Can you work these out from the model? Positions are in its coordinate system, mm. A direction names the side the tool comes from. Give positions to 0.01 mm unless a question says otherwise; leave off trailing zeros. Loops run counter-clockwise (first coordinate to the right, second up) from the corner with the lowest first, then second, coordinate; pieces in that order, holes last. Notation, with made-up numbers: (-36.5, 4.25) - (12.5, 4.25) arc R33 ccw to (12.5, 33.25) - close; hole circle Ø3 at (67, 45.5). An arc over 180 degrees is marked (long way). Write item = value, one per line.
from build123d import *

# Parameters (mm, degrees)
F1_DEPTH  = 9
F2_W      = 42.22
F2_H      = 1.875
F3_DEPTH  = 1
F4_W      = 10
F4_H      = 9
F5_DEPTH  = 10
F6_R      = 9.99999
F7_R      = 4.5
F8_DEPTH  = 25
F10_DEPTH = 5
F12_DEPTH = 25


# Not quite as in the source:
# - a fillet or chamfer is up to 0.001 mm smaller than in the source, because OpenCascade refuses the exact size


with BuildPart() as f1:
    # F0 (on Front) → F1 (new body)
    with BuildSketch(Plane.XZ):
        Polygon((30, 3.7309644414), (0, 3.7309644414), (-30, 3.7309644414), (-40, 18.7309644414), (-45, 18.7309644414), (-40, -1.2690355586), (-45, -11.2690355586), (-30, -6.2690355586), (0, -6.2690355586), (30, -6.2690355586), (45, -11.2690355586), (40, -1.2690355586), (45, 18.7309644414), (40, 18.7309644414), align=None)
    extrude(amount=F1_DEPTH)

    # F2 (on face) → F3 (cut)
    with BuildSketch(Plane.XY.offset(3.7309644414)):
        Polygon((21.11, -8.25), (25, -4.5), (21.11, -4.5), (21.11, -6.375), align=None)
        Polygon((21.11, -4.5), (25, -4.5), (21.11, -0.75), (21.11, -2.625), align=None)
        with Locations((0, -5.4375)):
            Rectangle(F2_W, F2_H)
        with Locations((0, -3.5625)):
            Rectangle(F2_W, F2_H)
        Polygon((-21.11, -6.375), (-21.11, -4.5), (-25, -4.5), (-21.11, -8.25), align=None)
        Polygon((-25, -4.5), (-21.11, -4.5), (-21.11, -2.625), (-21.11, -0.75), align=None)
    extrude(amount=-F3_DEPTH, mode=Mode.SUBTRACT)

    # F4 (on face) → F5 (join)
    with BuildSketch(Plane(origin=(0, 0, -6.2690355586), x_dir=(1, 0, 0), z_dir=(0, 0, -1))):
        with Locations((0, 4.5)):
            Rectangle(F4_W, F4_H)
    extrude(amount=F5_DEPTH)

    # F6 (radius 10 in the source; OpenCascade refuses exactly that, so slightly less here)
    f6_edges = [f1.edges().sort_by_distance(p)[0] for p in [
        (5, -4.5, -6.269036),
        (-5, -4.5, -6.269036),
    ]]
    fillet(f6_edges, radius=F6_R)

    # F7 (on face) → F8 (join)
    with BuildSketch(Plane(origin=(0, 0, -16.2690355586), x_dir=(1, 0, 0), z_dir=(0, 0, -1))):
        with Locations((0, 4.5)):
            Circle(F7_R)
    extrude(amount=F8_DEPTH)

    # F9 (on face) → F10 (join)
    with BuildSketch(Plane(origin=(0, 0, -41.2690355586), x_dir=(1, 0, 0), z_dir=(0, 0, -1))):
        Polygon((-10, 0), (0, 0), (10.0785335526, 0), (10.0785335526, 9), (0, 9), (-10, 9), align=None)
    extrude(amount=F10_DEPTH)

    # F11 (on face) → F12 (cut)
    with BuildSketch(Plane.XZ.offset(9)):
        Polygon((-10, -41.2690355586), (-10, -42.9390355586), (-4.5407158323, -41.2690355586), align=None)
        Polygon((10.0785335526, -41.2690355586), (4.5102024451, -41.2690355586), (10.0785335526, -42.9390355586), align=None)
    extrude(amount=-F12_DEPTH, mode=Mode.SUBTRACT)


solid = f1.part
Q1. For pin 1 (2 mm diameter, centred on y = -3, z = -30, fed in from -X); pin 2 (3 mm diameter, centred on y = -6, z = -20.5, fed in from +X); pin 3 (1.1 mm diameter, centred on y = -7, z = 3, fed in from +X); pin 4 (10 mm diameter, centred on x = 30, z = 6.5, fed in from +Y), each with a flat end and sliding along its axis, tell me the tip position at first contact or that it passes through.
Output:
pin_1 = -4.47
pin_2 = 4.5
pin_3 = 41.2
pin_4 = 0
Q2. Imagine slicing it at D-D, the plane x = 36. Write out the boundary of the cut face in (y, z).
Output:
outline = (-9, -8.27) - (0, -8.27) - (0, 12.73) - (-9, 12.73) - close
Q3. We'd pull the mould along Z, two halves only. Please class faces 1 (the flat face through (-7.309, -4.563, -42.116)), 2 (the flat face through (-42.465, -4.437, -6.199)), 3 (the flat face through (-34.93, -4.437, 11.126)), 4 (the flat face through (-1, 0, 1)): released by +Z, released by -Z, zero draft, split by the parting line, or undercut.
Output:
face_1 = undercut
face_2 = undercut
face_3 = released by +Z
face_4 = zero draft
Q4. Imagine slicing it at A-A, the plane x = -19. Write out the boundary of the cut face in (y, z) (3 decimals).
Output:
outline = (-9, -6.269) - (0, -6.269) - (0, 3.731) - (-2.625, 3.731) - (-2.625, 2.731) - (-6.375, 2.731) - (-6.375, 3.731) - (-9, 3.731) - close
Q5. Imagine slicing it at B-B, the plane x = -9. Write out the boundary of the cut face in (y, z) (3 decimals), then the cut area to 3 significant figures.
Output:
outline = (-9, -46.269) - (0, -46.269) - (0, -42.633) - (-9, -42.633) - close; (-9, -8.269) - (0, -8.269) - (0, 3.731) - (-2.625, 3.731) - (-2.625, 2.731) - (-6.375, 2.731) - (-6.375, 3.731) - (-9, 3.731) - close
area = 137 mm2
Q6. Which directions (+Z, -Z, +X, -X, +Y, -Y) give clear straight access to the entire face, cutting with the end or side of a thin tool? Please do faces 5 (the flat face through (4, -7, -41.269)), 6 (the flat face through (42.465, -4.437, 8.591)), 7 (the flat face through (-4.7, -4.5, -16.269)), 8 (the flat face through (35.07, -4.437, 11.336)), 9 (the flat face through (10.079, -4, -45)).
Output:
face_5 = +X
face_6 = +X, +Y, -Y
face_7 = -X
face_8 = +Z, +Y, -Y
face_9 = -Z, +X, +Y, -Y
Q7. I need wall thicknesses on L1, parallel to Z at x = -2.5, y = -8.5; L2, parallel to Z at x = 24, y = -3.5; L3, parallel to Z at x = 20, y = -4.5. Which ranges of each line are inside material? Lowest first, please.
Output:
L1 = -46.27 to -41.27, -16.27 to 3.73
L2 = -6.27 to 3.73
L3 = -6.27 to 2.73
Q8. Imagine slicing it at C-C, the plane z = -4.5. Write out the boundary of the cut face in (x, y).
Output:
outline = (-41.62, -9) - (41.62, -9) - (41.62, 0) - (-41.62, 0) - close
